from build123d import *

# Parameters (mm, degrees)
SKETCH_1_R          = 12
EXTRUDE_1_DEPTH     = 4
SKETCH_2_R          = 12
SKETCH_2_R_2        = 10
EXTRUDE_2_DEPTH     = 20
SKETCH_4_R          = 1.5
CUT_EXTRUDE_1_DEPTH = 25
SKETCH_6_R          = 2.5
CUT_EXTRUDE_2_DEPTH = 3.5
SKETCH_7_R          = 1
CUT_EXTRUDE_3_DEPTH = 25


with BuildPart() as part:
    # 스케치1 → 보스-돌출1 (new body)
    with BuildSketch(Plane.XY):
        Circle(SKETCH_1_R)
    extrude(amount=EXTRUDE_1_DEPTH)

    # 스케치2 → 보스-돌출2 (add)
    with BuildSketch(Plane.XY.offset(4)):
        Circle(SKETCH_2_R)
        Circle(SKETCH_2_R_2, mode=Mode.SUBTRACT)
    extrude(amount=EXTRUDE_2_DEPTH)

    # 스케치4 → 컷-돌출1 (cut, through all)
    with BuildSketch(Plane(origin=(0, 0, 0), x_dir=(-1, 0, 0), z_dir=(0, 0, -1))):
        Circle(SKETCH_4_R)
    extrude(amount=-CUT_EXTRUDE_1_DEPTH, mode=Mode.SUBTRACT)

    # 스케치6 → 컷-돌출2 (cut)
    with BuildSketch(Plane(origin=(0, 0, 0), x_dir=(-1, 0, 0), z_dir=(0, 0, -1))):
        Circle(SKETCH_6_R)
    extrude(amount=-CUT_EXTRUDE_2_DEPTH, mode=Mode.SUBTRACT)

    # 스케치7 → 컷-돌출3 (cut, through all)
    with BuildSketch(Plane(origin=(0, 0, 0), x_dir=(-1, 0, 0), z_dir=(0, 0, -1))):
        with Locations((-5, 0)):
            Circle(SKETCH_7_R)
        with Locations((5, 0)):
            Circle(SKETCH_7_R)
    extrude(amount=-CUT_EXTRUDE_3_DEPTH, mode=Mode.SUBTRACT)


solid = part.part
Model file for the job. Use its own axes, mm. A direction names the side the tool comes from. Round coordinates to 2 decimals unless told otherwise and drop trailing zeros. Order: outer loops, then holes, each group sorted by start corner. A loop starts at its lowest first (then second) coordinate and runs counter-clockwise, first axis right, second up. Notation, with made-up numbers: M 25,-5.5 L 79,-5.5 A25 ccw 79,10.5 Z; hole C 43,13 d1. An arc over 180 degrees is marked long. Write each question's results on one line, items separated by ' | '. Start each with the question number.
(1) Probe probe 1 along Y at (x, z) = (0, 2.2); probe 2 along Z at (x, y) = (-3.5, -6.25); probe 3 along Y at (x, z) = (0, 3.7). List the from-to ranges inside material, lowest first. Write a range as from..to.
(2) Drop flat-ended pins along their axis: pin 1 (2 mm diameter, centred on x = 6, z = 21.5, fed in from +Y); pin 2 (1.5 mm diameter, centred on x = -1, y = 1, fed in from -Z); pin 3 (1.8 mm diameter, centred on x = 5, y = 0, fed in from -Z); pin 4 (6.5 mm diameter, centred on x = 0, y = 0, fed in from +Z). Give the stop position or say it passes through.
(3) Saw through at D-D, the plane z = 11. Give the cut face in (x, y), then the cut area to 3 significant figures.
(4) Two-plate mould, pull along Y, no slides. Class faces 4 (the face through (-11.99, 0.53, 11.83)), 5 (the face through (5.8, -0.6, 2)), 6 (the face through (0, 3, 0)): pulls with the +Y half, pulls with the -Y half, needs draft (parallel to the pull), parting line crosses it, or undercut.
(5) Saw through at B-B, the plane x = 0. Give the cut face in (y, z).
(6) Which spindle directions (+Z, -Z, +X, -X, +Y, -Y) get a long thin tool onto all of the face, cutting with end or side? Do faces 1 (the face through (1.5, 0.07, 3.75)), 2 (the face through (-2.17, -9.76, 13.86)), 3 (the face through (0, -2, 3.5)). Say none if no direction does.
(7) Saw through at C-C, the plane y = -9.5. Give the cut face in (x, z), then the cut area to 3 significant figures.
(8) Saw through at A-A, the plane y = 0. Give the cut face in (x, z), then the cut area to 3 significant figures.
Established:
1) probe 1: y = -12..-2.5, 2.5..12 | probe 2: z = 0..4 | probe 3: y = -12..-1.5, 1.5..12
2) pin 1: stops at y = 10.91 | pin 2: stops at z = 3.5 | pin 3: passes through | pin 4: stops at z = 4
3) outline: C 0,0 d24; hole C 0,0 d20 | area: 138 mm^2
4) face 4: parting line crosses it | face 5: undercut | face 6: needs draft
5) outline: M -12,0 L -2.5,0 L -2.5,3.5 L -1.5,3.5 L -1.5,4 L -10,4 L -10,24 L -12,24 Z; M 1.5,3.5 L 2.5,3.5 L 2.5,0 L 12,0 L 12,24 L 10,24 L 10,4 L 1.5,4 Z
6) face 1: +Z, -Z | face 2: +Z | face 3: -Z
7) outline: M -7.33,0 L 7.33,0 L 7.33,24 L 3.12,24 L 3.12,4 L -3.12,4 L -3.12,24 L -7.33,24 Z | area: 227 mm^2
8) outline: M -12,0 L -6,0 L -6,4 L -10,4 L -10,24 L -12,24 Z; M -4,0 L -2.5,0 L -2.5,3.5 L -1.5,3.5 L -1.5,4 L -4,4 Z; M 1.5,3.5 L 2.5,3.5 L 2.5,0 L 4,0 L 4,4 L 1.5,4 Z; M 6,0 L 12,0 L 12,24 L 10,24 L 10,4 L 6,4 Z | area: 141 mm^2
